Check sheet for the modelled part. Datum: model origin and axes. Units: mm. A direction names the side the tool comes from. Round coordinates to 2 decimals unless told otherwise and drop trailing zeros. Loops run counter-clockwise (first coordinate to the right, second up) from the corner with the lowest first, then second, coordinate; pieces in that order, holes last. Notation, with made-up numbers: (16.5, 67) -> (38.5, 67) arc R30 cw to (38.5, 99) -> close; hole circle Ø3 at (42.25, 34). An arc over 180 degrees is marked (long way). Return JSON: item names as keys, results as strings.
from build123d import *

# Parameters (mm, degrees)
ESQUISSE1_W = 12
ESQUISSE1_H = 10


with BuildPart() as part:
    # Balayage1: sweep along a path in Esquisse2
    with BuildLine(Plane(origin=(0, 0, 0), x_dir=(0, 0, -1), z_dir=(1, 0, 0))) as balayage1_path:
        Line((0, 0), (0, -37.597886471))
        ThreePointArc((0, -37.597886471), (-20.015041061, -54.69234646), (-33.767997639, -32.249561064))
        Line((-33.767997639, -32.249561064), (-12.263031239, 33.935919993))
    # Esquisse1 → Balayage1 (sweep)
    with BuildSketch(Plane(origin=(0, 0, 0), x_dir=(1, 0, 0), z_dir=(0, 1, 0))):
        Rectangle(ESQUISSE1_W, ESQUISSE1_H)
    sweep(path=balayage1_path.line)


solid = part.part
Q1. Section check B-B (y = -6). Record the boundary of the cut face in (x, z), then the cut area to 3 significant figures.
Results list:
{"outline": "(-6, -5) -> (6, -5) -> (6, 5) -> (-6, 5) -> close; (-6, 19.98) -> (6, 19.98) -> (6, 30.5) -> (-6, 30.5) -> close", "area": "246 mm^2"}
Q2. Section check C-C (x = -4.25). Record the boundary of the cut face in (y, z).
Results list:
{"outline": "(-37.6, -5) -> (0, -5) -> (0, 5) -> (-37.6, 5) arc R12.31 cw (long way) to (-33.79, 29.01) -> (32.39, 7.51) -> (35.48, 17.02) -> (-30.7, 38.52) arc R22.31 ccw (long way) to start"}
Q3. Tool access check on faces 1 (the flat face through (0, -19, 5)), 2 (the flat face through (0.08, 2.85, 27.62)). Record the directions out of +Z, -Z, +X, -X, +Y, -Y that give a thin tool (end or side, any length) a straight path to the whole face; none if there is none.
Results list:
{"face 1": "+X, -X, +Y", "face 2": "+Z, +X, -X, +Y"}
Q4. Section check A-A (z = 8.5). Record the boundary of the cut face in (x, y).
Results list:
{"outline": "(-6, -58.09) -> (6, -58.09) -> (6, -46.19) -> (-6, -46.19) -> close; (-6, 29.34) -> (6, 29.34) -> (6, 32.71) -> (-6, 32.71) -> close"}
Q5. Section check D-D (y = -51). Record the boundary of the cut face in (x, z), then the cut area to 3 significant figures.
Results list:
{"outline": "(-6, -0.53) -> (6, -0.53) -> (6, 35.14) -> (-6, 35.14) -> close", "area": "428 mm^2"}
Q6. Go/stop test with flat-tipped pins: pin 1 (2 mm diameter, centred on x = 3.5, z = 19.5, fed in from -Y); pin 2 (3 mm diameter, centred on x = -1.5, z = 2, fed in from +Y); pin 3 (2 mm diameter, centred on x = -0.5, y = -50, fed in from -Z). Record where each tip stops, or that it passes through.
Results list:
{"pin 1": "y = -59.87", "pin 2": "y = 0", "pin 3": "z = -1.87"}
Q7. Material ranges on line 1 (Z direction, x = 2.75, y = -46); line 2 (Z direction, x = 4, y = -39); line 3 (Z direction, x = -2, y = 9.5), recorded low to high.
Results list:
{"line 1": "-3.36 to 8.31, 26.3 to 37.97", "line 2": "-4.96 to 5.08, 29.53 to 39.57", "line 3": "14.95 to 25.46"}
Q8. Draft check along Z on faces 3 (the flat face through (0, 0, 0)), 4 (the flat face through (0.084, 33.958, 12.33)), 5 (the flat face through (-0.08, -0.24, 18.11)). Enter one of: released by +Z, released by -Z, zero draft, split by the parting line, or undercut.
Results list:
{"face 3": "zero draft", "face 4": "released by -Z", "face 5": "undercut"}
